```python
from build123d import *

# Parameters (mm, degrees)
BOSS_EXTRUDE1_DEPTH = 20
SKETCH2_R           = 1.5
CUT_EXTRUDE1_DEPTH  = 5
FILLET1_R           = 2
SKETCH3_W           = 30
SKETCH3_H           = 20
CUT_EXTRUDE2_DEPTH  = 10


with BuildPart() as part:
    # Sketch1 → Boss-Extrude1 (new, symmetric)
    with BuildSketch(Plane(origin=(0, 0, 0), x_dir=(1, 0, 0), z_dir=(0, 1, 0))):
        Polygon((-110, 0), (-80, 40), (80, 40), (110, 0), (103, 0), (77.5, 34), (-77.5, 34), (-103, 0), align=None)
    extrude(amount=BOSS_EXTRUDE1_DEPTH, both=True)

    # Sketch2 → Cut-Extrude1 (cut)
    with BuildSketch(Plane(origin=(0, 20, 0), x_dir=(1, 0, 0), z_dir=(0, 1, 0))):
        with Locations(Location((-104, 3, 0), (0, 0, 270))):
            Circle(SKETCH2_R)
        with Locations(Location((-77, 37, 0), (0, 0, 270))):
            Circle(SKETCH2_R)
        with Locations(Location((-7, 37, 0), (0, 0, 270))):
            Circle(SKETCH2_R)
        with Locations(Location((7, 37, 0), (0, 0, 90))):
            Circle(SKETCH2_R)
        with Locations(Location((77, 37, 0), (0, 0, 90))):
            Circle(SKETCH2_R)
        with Locations(Location((104, 3, 0), (0, 0, 90))):
            Circle(SKETCH2_R)
    extrude(amount=-CUT_EXTRUDE1_DEPTH, mode=Mode.SUBTRACT)

    # Fillet1
    fillet1_edges = [part.edges().sort_by_distance(p)[0] for p in [
        (-80, 0, -40),
        (80, 0, -40),
    ]]
    fillet(fillet1_edges, radius=FILLET1_R)

    # Sketch3 → Cut-Extrude2 (cut)
    with BuildSketch(Plane(origin=(-70.4, 0, -52.8), x_dir=(-0.5999999999999998, 0, 0.8000000000000003), z_dir=(-0.8000000000000004, 0, -0.5999999999999998))):
        with Locations((51, -5)):
            Rectangle(SKETCH3_W, SKETCH3_H)
    extrude(amount=-CUT_EXTRUDE2_DEPTH, mode=Mode.SUBTRACT)


solid = part.part
```
Check sheet for the modelled part. Datum: model origin and axes. Units: mm. A direction names the side the tool comes from. Give positions to 0.01 mm unless a question says otherwise; leave off trailing zeros. Write each loop counter-clockwise with the first axis right and the second up, starting at its lowest first coordinate (ties: lowest second). Pieces come first, ordered by that corner, then holes. Notation, with made-up numbers: (-3, 49) -> (40, 49) arc R30 cw to (40, 83) -> close; hole circle Ø8 at (82, 60). An arc over 180 degrees is marked (long way). Use CSV: the item, a comma, the result in double quotes. Start each with the question number.
Q1. Cross-section at C-C on z = -11. Enter the section's corners in (x, y).
Q2. Release check for a two-part mould opening along Y. For faces 1 (the flat face through (-89.791, -5.14, -22.344)), 2 (the flat face through (1, 20, -35)), 3 (the flat face through (-87.238, 0.28, -21.016)) record: +Y half, -Y half, draft (parallel to the pull), parting line (faces both ways), or undercut.
Q3. Cross-section at D-D on x = -37.5. Enter the section's corners in (y, z), and give its area (3 significant figures).
Q4. Scan lines: line 1 along Z through (x, y) = (77, 17.15); line 2 along X through (y, z) = (18, -37); line 3 along X through (y, z) = (16, -3). Record each from-to range of solid material in increasing order.
Q5. Cross-section at B-B on y = 13. Enter the section's corners in (x, z), and give its area (3 significant figures).
Q6. Cross-section at A-A on z = -32. Enter the section's corners in (x, y).
Q7. Tool access check on faces 4 (the flat face through (-99, -15, -11)), 5 (the flat face through (1, 0, -34)), 6 (the flat face through (-106, 13, 0)). Record the directions out of +Z, -Z, +X, -X, +Y, -Y that give a thin tool (end or side, any length) a straight path to the whole face; none if there is none.
Q8. Depth check by flat-ended pin: P1, Ø2.5, axis at x = 104, z = -3, coming from the +Y side; P2, Ø1, axis at x = -69, y = -7, coming from the +Z side; P3, Ø6, axis at x = 80.5, y = -12, coming from the +Z side. Enter the tip coordinate at first touch or a pass-through.
Working result:
1,outline,"(-101.75, -20) -> (-94.75, -20) -> (-94.75, -15) -> (-101.75, -15) -> close; (-101.75, 5) -> (-94.75, 5) -> (-94.75, 20) -> (-101.75, 20) -> close; (94.75, -20) -> (101.75, -20) -> (101.75, 20) -> (94.75, 20) -> close"
2,face 1,"undercut"
2,face 2,"+Y half"
2,face 3,"draft"
3,outline,"(-20, -40) -> (20, -40) -> (20, -34) -> (-20, -34) -> close"
3,area,"240 mm^2"
4,line 1,"z = -40 to -38.5, -35.5 to -34"
4,line 2,"x = -82.25 to -78.5, -75.5 to -8.5, -5.5 to 5.5, 8.5 to 75.5, 78.5 to 82.25"
4,line 3,"x = -107.75 to -105.5, -102.5 to -100.75, 100.75 to 102.5, 105.5 to 107.75"
5,outline,"(-110, 0) -> (-80.6, -39.2) arc R2 ccw to (-79, -40) -> (79, -40) arc R2 ccw to (80.6, -39.2) -> (110, 0) -> (103, 0) -> (77.5, -34) -> (-77.5, -34) -> (-103, 0) -> close"
5,area,"1,460 mm^2"
6,outline,"(-86, -20) -> (-79, -20) -> (-79, 20) -> (-86, 20) -> close; (79, -20) -> (86, -20) -> (86, 20) -> (79, 20) -> close"
7,face 4,"+Z, -X"
7,face 5,"+Z, +Y, -Y"
7,face 6,"+Z, +X, -X, +Y, -Y"
8,P1,"stops at y = 15"
8,P2,"stops at z = -34"
8,P3,"stops at z = -26"
